Autodesk Inventor part; units mm, degrees
ref_plane "YZ Plane" through (0, 0, 0) normal (1, 0, 0) x (0, 1, 0)
ref_plane "XZ Plane" through (0, 0, 0) normal (0, 1, 0) x (-1, 0, 0)
ref_plane "XY Plane" through (0, 0, 0) normal (0, 0, 1) x (1, 0, 0)
sketch "Sketch1" plane through (0, 0, 0) normal (0, 1, 0) x (-1, 0, 0)
  line L0 (2.2807, -2.5252) -> (-23.1193, -2.5252)
  line L1 (-23.1193, -2.5252) -> (-23.1193, 48.2748)
  line L2 (-23.1193, 48.2748) -> (2.2807, 48.2748)
  line L3 (2.2807, 48.2748) -> (2.2807, -2.5252)
  line L4 (-19.9443, 0.6498) -> (-0.8943, 0.6498)
  line L5 (-0.8943, 0.6498) -> (-0.8943, 45.0998)
  line L6 (-0.8943, 45.0998) -> (-19.9443, 45.0998)
  line L7 (-19.9443, 45.0998) -> (-19.9443, 0.6498)
  point P0 (0, 0)
  dimension "d0" = 25.4
  dimension "d1" = 50.8
  dimension "d2" = 3.175
extrude "Extrusion1" add sketch "Sketch1" along normal blind 762
sketch "Sketch3" plane through (-2.2807, 0, 48.2748) normal (0, 0, 1) x (1, 0, 0)
  line L0 (22.225, 0) -> (3.175, 0) construction
  line L1 (12.7, 0) -> (12.7, 12.7) construction
  line L2 (12.7, 12.7) -> (12.7, 38.1) construction
  line L3 (12.7, 38.1) -> (12.7, 63.5) construction
  circle A0 centre (12.7, 63.5) radius 2.5797
  circle A1 centre (12.7, 38.1) radius 2.5797
  circle A2 centre (12.7, 12.7) radius 2.5797
  line L4 (12.7, 685.8) -> (12.7, 673.1) construction
  circle A3 centre (12.7, 673.1) radius 2.5797
  line L5 (12.7, 673.1) -> (12.7, 647.7) construction
  line L6 (12.7, 647.7) -> (12.7, 622.3) construction
  circle A4 centre (12.7, 647.7) radius 2.5797
  circle A5 centre (12.7, 622.3) radius 2.5797
  point P0 (2.2807, 0)
  dimension "d19" = 12.7
  dimension "d20" = 25.4
  dimension "d21" = 25.4
  dimension "d22" = 5.1594
  dimension "d23" = 5.1594
  dimension "d24" = 5.1594
  dimension "d38" = 12.7
  dimension "d39" = 5.1594
  dimension "d40" = 25.4
  dimension "d41" = 25.4
  dimension "d42" = 5.1594
  dimension "d43" = 5.1594
extrude "Extrusion3" cut sketch "Sketch3" against normal blind 762
sketch "Sketch4" plane through (23.1193, 0, 48.2748) normal (1, 0, 0) x (0, 0, -1)
  line L0 (3.175, 762) -> (47.625, 762) construction
  line L1 (25.4, 762) -> (25.4, 736.6) construction
  point P0 (48.2748, 0)
  dimension "d44" = 25.4
sketch "Sketch5" plane through (-2.2807, 0, -2.5252) normal (-1, 0, 0) x (0, 0, 1)
  circle A0 centre (25.4, 12.7) radius 2.5797
  line L0 (50.8, 0) -> (50.8, 762)
  circle A1 centre (25.4, 38.1) radius 2.5797 construction
  line L1 (50.8, 38.1) -> (38.1, 38.1) construction
  circle A2 centre (25.4, 63.5) radius 2.5797 construction
  line L2 (50.8, 63.5) -> (38.1, 63.5) construction
  circle A3 centre (38.1, 63.5) radius 2.5797
  circle A4 centre (38.1, 38.1) radius 2.5797
  circle A5 centre (38.1, 12.7) radius 2.5797
  line L3 (38.1, 12.7) -> (50.8, 12.7) construction
  circle A6 centre (25.4, 622.3) radius 2.5797 construction
  line L4 (50.8, 622.3) -> (38.1, 622.3) construction
  circle A7 centre (25.4, 647.7) radius 2.5797 construction
  line L5 (50.8, 647.7) -> (38.1, 647.7) construction
  circle A8 centre (25.4, 673.1) radius 2.5797 construction
  line L6 (50.8, 673.1) -> (38.1, 673.1) construction
  circle A9 centre (38.1, 647.7) radius 2.5797
  circle A10 centre (38.1, 622.3) radius 2.5797
  circle A11 centre (38.1, 673.1) radius 2.5797
  point P0 (2.5252, 0)
  dimension "d46" = 12.7
  dimension "d47" = 12.7
  dimension "d48" = 5.1594
  dimension "d49" = 5.1594
  dimension "d50" = 5.1594
  dimension "d51" = 12.7
  dimension "d52" = 12.7
  dimension "d53" = 12.7
  dimension "d54" = 5.1594
  dimension "d55" = 5.1594
  dimension "d56" = 5.1594
extrude "Extrusion4" cut sketch "Sketch5" against normal blind 762 contours A3 | A4 | A5 | A9 | A10 | A11
sketch "Sketch6" plane through (-2.2807, 0, -2.5252) normal (-1, 0, 0) x (0, 0, 1)
  line L0 (47.625, 762) -> (3.175, 762) construction
  line L1 (25.4, 762) -> (25.4, 736.6) construction
  circle A0 centre (25.4, 736.6) radius 14.2875
  point P0 (2.5252, 0)
  dimension "d59" = 25.4
  dimension "d60" = 28.575
extrude "Extrusion5" cut sketch "Sketch6" against normal blind 304.8
sketch "Sketch7" plane through (-2.2807, 0, -2.5252) normal (-1, 0, 0) x (0, 0, 1)
  circle A0 centre (38.1, 12.7) radius 2.5797 construction
  line L0 (38.1, 12.7) -> (38.1, 114.3) construction
  line L1 (38.1, 12.7) -> (38.1, 190.5) construction
  line L2 (38.1, 190.5) -> (12.7, 190.5) construction
  line L3 (38.1, 114.3) -> (12.7, 114.3) construction
  circle A1 centre (38.1, 190.5) radius 2.5797
  circle A2 centre (12.7, 190.5) radius 2.5797
  circle A3 centre (38.1, 114.3) radius 2.5797
  circle A4 centre (12.7, 114.3) radius 2.5797
  point P0 (2.5252, 0)
  dimension "d63" = 101.6
  dimension "d64" = 177.8
  dimension "d65" = 25.4
  dimension "d66" = 25.4
  dimension "d67" = 5.1594
  dimension "d68" = 5.1594
  dimension "d69" = 5.1594
  dimension "d70" = 5.1594
extrude "Extrusion6" cut sketch "Sketch7" against normal blind 50.8
properties part number "30in 1x1 Beam"
The model under review builds one solid part; all positions refer to its coordinate system, in mm. A direction names the side the tool comes from. Round coordinates to 2 decimals unless told otherwise and drop trailing zeros. Write each loop counter-clockwise with the first axis right and the second up, starting at its lowest first coordinate (ties: lowest second). Pieces come first, ordered by that corner, then holes.
(1) We need section B-B on y = 440. Give the boundary of the cut face in (x, z), and give its area (3 significant figures).
(2) Mouldability with a two-part tool opening along Z and no side actions: class faces 3 (the flat face through (10, 376, -2.525)), 4 (the flat face through (0.894, 376, 23)), 5 (the flat face through (23.119, 376, 23)) as +Z half, -Z half, draft (parallel to the pull), parting line (faces both ways), or undercut.
(3) Insertion check: pin 1 (4 mm diameter, centred on y = 622.3, z = 35.57, fed in from -X); pin 2 (8.5 mm diameter, centred on x = 10.42, y = 38.1, fed in from -Z). Each pin has a flat end and moves straight along its axis. Give the tip position at first contact, or say it passes through.
(4) We need section A-A on y = 736.6. Give the boundary of the cut face in (x, z), and give its area (3 significant figures).
(5) Wall thickness on L1, parallel to X at y = 72, z = 12; L2, parallel to Z at x = 16.5, y = 212.5; L3, parallel to X at y = 673.1, z = 46.1: over which ranges is each line inside the solid? List them lowest first.
(6) Machinability: for faces 1 (the flat face through (19.944, 376, 23)), 2 (the cylindrical face through (21.51, 722.65, 19.78)), which of the approach directions +Z, -Z, +X, -X, +Y, -Y give a long, thin tool a straight path to every point of the face, cutting with its end or side? Answer none if there is none.
Findings below:
1. outline: (-2.28, -2.53) - (23.12, -2.53) - (23.12, 48.27) - (-2.28, 48.27) - close; hole (0.89, 0.65) - (19.94, 0.65) - (19.94, 45.1) - (0.89, 45.1) - close
1. area: 444 mm2
2. face 3: -Z half
2. face 4: undercut
2. face 5: draft
3. pin 1: passes through
3. pin 2: stops at z = -2.53
4. outline: (-2.28, -2.53) - (23.12, -2.53) - (23.12, 8.59) - (19.94, 8.59) - (19.94, 0.65) - (0.89, 0.65) - (0.89, 8.59) - (-2.28, 8.59) - close; (-2.28, 37.16) - (0.89, 37.16) - (0.89, 45.1) - (19.94, 45.1) - (19.94, 37.16) - (23.12, 37.16) - (23.12, 48.27) - (-2.28, 48.27) - close
4. area: 262 mm2
5. L1: x = -2.28 to 0.89, 19.94 to 23.12
5. L2: z = -2.53 to 0.65, 45.1 to 48.27
5. L3: x = -2.28 to 7.84, 13 to 23.12
6. face 1: +Y, -Y
6. face 2: +X, -X
